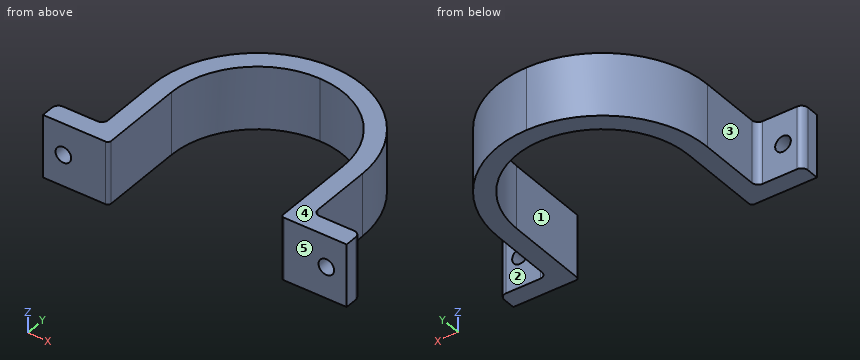
from build123d import *

# Parameters (mm, degrees)
PAD_DEPTH                  = 10
SKETCH001_R                = 2.5
POCKET_DEPTH               = 293.638056
SKETCH001_MIRRORED001_2_R  = 2.5
POCKET_MIRRORED001_2_DEPTH = 293.638056


with BuildPart() as part:
    # Sketch → Pad (new body, symmetric)
    with BuildSketch(Plane.XY):
        with BuildLine():
            ThreePointArc((27.5, 27.5), (19.445436, 46.945436), (0, 55))
            Line((0, 55), (0, 61))
            ThreePointArc((33.5, 27.5), (23.688077, 51.188077), (0, 61))
            Line((33.5, 27.5), (33.5, 8))
            ThreePointArc((33.5, 8), (34.085786, 6.585786), (35.5, 6))
            Line((46.5, 6), (35.5, 6))
            ThreePointArc((48.5, 4), (47.914214, 5.414214), (46.5, 6))
            Line((48.5, 0), (48.5, 4))
            Line((28.5, 0), (48.5, 0))
            ThreePointArc((27.5, 1), (27.792893, 0.292893), (28.5, 0))
            Line((27.5, 27.5), (27.5, 1))
        make_face()
    pad = extrude(amount=PAD_DEPTH, both=True)

    # Mirrored: Pad across Sketch V_Axis
    add(pad.mirror(Plane(origin=(0, 0, 0), x_dir=(0, 0, 1), z_dir=(1, 0, 0))))

    # Sketch001 → Pocket (cut, through all)
    with BuildSketch(Plane.XZ):
        with Locations((42, 0)):
            Circle(SKETCH001_R)
    pocket = extrude(amount=-POCKET_DEPTH, mode=Mode.SUBTRACT)

    # Sketch001 Mirrored001 2 → Pocket Mirrored001 2 (cut, through all)
    with BuildSketch(Plane(origin=(0, 0, 0), x_dir=(1, 0, 0), z_dir=(0, 1, 0))):
        with Locations((42, 0)):
            Circle(SKETCH001_MIRRORED001_2_R)
    pocket_mirrored001_2 = extrude(amount=POCKET_MIRRORED001_2_DEPTH, mode=Mode.SUBTRACT)

    # Mirrored002: Pocket, Pocket Mirrored001 2 across Sketch001 V_Axis
    add(pocket.mirror(Plane(origin=(0, 0, 0), x_dir=(0, -1, 0), z_dir=(1, 0, 0))), mode=Mode.SUBTRACT)
    add(pocket_mirrored001_2.mirror(Plane(origin=(0, 0, 0), x_dir=(0, -1, 0), z_dir=(1, 0, 0))), mode=Mode.SUBTRACT)


solid = part.part
Part model, mm, in its own coordinate system. Face numbers are marked on the shaded views. A direction names the side the tool comes from. Give positions to 0.01 mm unless a question says otherwise; leave off trailing zeros. Loops run counter-clockwise (first coordinate to the right, second up) from the corner with the lowest first, then second, coordinate; pieces in that order, holes last.
(1) Pin check, flat tips, straight feed: pin 1 (1.5 mm diameter, centred on x = -12, z = -6, fed in from +Y); pin 2 (10 mm diameter, centred on y = 13.5, z = 2, fed in from -X); pin 3 (1 mm diameter, centred on y = 19.5, z = -1.5, fed in from +X); pin 4 (3 mm diameter, centred on x = -42, z = 0, fed in from +Y). Stop position of each tip, or through.
Return value:
pin 1: stops at y = 59.05
pin 2: stops at x = -33.5
pin 3: stops at x = 33.5
pin 4: passes through
(2) Band-saw the part on A-A (x = 42). Write the cut outline in (y, z).
Return value:
outline: (0, -10) - (6, -10) - (6, -2.5) - (0, -2.5) - close; (0, 2.5) - (6, 2.5) - (6, 10) - (0, 10) - close
(3) Band-saw the part on B-B (z = 0). Write the cut outline in (x, y), and give its area (3 significant figures).
Return value:
outline: (-48.5, 0) - (-44.5, 0) - (-44.5, 6) - (-46.5, 6) arc R2 ccw to (-48.5, 4) - close; (-39.5, 0) - (-28.5, 0) arc R1 ccw to (-27.5, 1) - (-27.5, 27.5) arc R27.5 cw to (0, 55) arc R27.5 cw to (27.5, 27.5) - (27.5, 1) arc R1 ccw to (28.5, 0) - (39.5, 0) - (39.5, 6) - (35.5, 6) arc R2 cw to (33.5, 8) - (33.5, 27.5) arc R33.5 ccw to (0, 61) arc R33.5 ccw to (-33.5, 27.5) - (-33.5, 8) arc R2 cw to (-35.5, 6) - (-39.5, 6) - close; (44.5, 0) - (48.5, 0) - (48.5, 4) arc R2 ccw to (46.5, 6) - (44.5, 6) - close
area: 1,020 mm2
(4) Band-saw the part on C-C (y = 10). Write the cut outline in (x, z).
Return value:
outline: (-33.5, -10) - (-27.5, -10) - (-27.5, 10) - (-33.5, 10) - close; (27.5, -10) - (33.5, -10) - (33.5, 10) - (27.5, 10) - close
(5) Band-saw the part on D-D (z = -4.25). Write the cut outline in (x, y).
Return value:
outline: (-48.5, 0) - (-28.5, 0) arc R1 ccw to (-27.5, 1) - (-27.5, 27.5) arc R27.5 cw to (0, 55) arc R27.5 cw to (27.5, 27.5) - (27.5, 1) arc R1 ccw to (28.5, 0) - (48.5, 0) - (48.5, 4) arc R2 ccw to (46.5, 6) - (35.5, 6) arc R2 cw to (33.5, 8) - (33.5, 27.5) arc R33.5 ccw to (0, 61) arc R33.5 ccw to (-33.5, 27.5) - (-33.5, 8) arc R2 cw to (-35.5, 6) - (-46.5, 6) arc R2 ccw to (-48.5, 4) - close
(6) 3-axis set-ups, long thin cutter, end or side, ignore diameter. For the marked faces 1, 2, 3, 4 and 5: which of +Z, -Z, +X, -X, +Y, -Y reach the whole face in a straight line?
Return value:
face 1: +Z, -Z, -Y
face 2: +Z, -Z, +X, +Y
face 3: +Z, -Z, -X, +Y
face 4: +Z, +X, -X, +Y, -Y
face 5: +Z, -Z, +X, -X, -Y
(7) Drill centre lines: line 1 along Z through (x, y) = (-42, 1.8); line 2 along X through (y, z) = (9.5, -3.25); line 3 along X through (y, z) = (4, 7.5). Where is each one in solid material? Low to high.
Return value:
line 1: z = -10 to -2.5, 2.5 to 10
line 2: x = -33.5 to -27.5, 27.5 to 33.5
line 3: x = -48.5 to -27.5, 27.5 to 48.5
